from build123d import *

# Parameters (mm, degrees)
EXTRUDE_START       = -15
SKETCH_1_R          = 17
EXTRUDE_1_DEPTH     = 35
SKETCH_2_R          = 10
EXTRUDE_2_DEPTH     = 47
FILLET_3_R          = 3
FILLET_4_R          = 20
SKETCH_4_W          = 20
SKETCH_4_H          = 21.133558335
CUT_EXTRUDE_2_DEPTH = 35
SKETCH_5_R          = 4
CUT_EXTRUDE_3_DEPTH = 35
CUT_EXTRUDE_START   = 20
SKETCH_6_W          = 15
SKETCH_6_H          = 20.573480962
CUT_EXTRUDE_4_DEPTH = 4
CUT_EXTRUDE_START_2 = -20
SKETCH_7_W          = 20
SKETCH_7_H          = 18.159164137
CUT_EXTRUDE_5_DEPTH = 4
SKETCH_8_R          = 4
CUT_EXTRUDE_6_DEPTH = 35


with BuildPart() as part:
    # Эскиз1 → Вытянуть1 (new body)
    with BuildSketch(Plane(origin=(0, 0, 0), x_dir=(1, 0, 0), z_dir=(0, 1, 0)).offset(EXTRUDE_START)):
        with Locations(Location((0, 0, 0), (0, 0, 270))):
            Circle(SKETCH_1_R)
    extrude(amount=EXTRUDE_1_DEPTH)

    # Эскиз2 → Вытянуть2 (add)
    with BuildSketch(Plane.XZ.offset(15)):
        with Locations(Location((0, 0, 0), (0, 0, 90))):
            Circle(SKETCH_2_R)
    extrude(amount=EXTRUDE_2_DEPTH)

    # Скругление3
    fillet_3_edges = [part.edges().sort_by_distance(p)[0] for p in [
        (0, 20, -17),
    ]]
    fillet(fillet_3_edges, radius=FILLET_3_R)

    # Скругление4
    # the kernel refuses this fillet: 20 mm, written as the material it adds along each edge
    with BuildSketch(Plane(origin=(0, -15, 0), x_dir=(0, 0, 1), z_dir=(1, 0, 0))) as fillet_4_piece_1:
        with BuildLine():
            CenterArc((30, 15.198684154), FILLET_4_R, 180, 49.458398126)
            Line((10, 15.198684154), (9.6, 15.198684154))
            Line((9.6, 15.198684154), (9.6, 0))
            Line((9.6, 0), (10, -0.4))
            ThreePointArc((10, -0.4), (13.5, -0.4), (16.74, -0.303973683))
            Line((16.74, -0.303973683), (17, 0))
        make_face()
    revolve(axis=Axis((0, -15, 0), (0, -1, 0)))

    # Эскиз4 → Вырез-Вытянуть2 (cut, symmetric)
    with BuildSketch(Plane.XY):
        with Locations((0, 10.566779168)):
            Rectangle(SKETCH_4_W, SKETCH_4_H)
    extrude(amount=CUT_EXTRUDE_2_DEPTH, both=True, mode=Mode.SUBTRACT)

    # Эскиз5 → Вырез-Вытянуть3 (cut, symmetric)
    with BuildSketch(Plane(origin=(0, 0, 0), x_dir=(0, 0, -1), z_dir=(1, 0, 0))):
        with Locations((0, 11.128860454)):
            Circle(SKETCH_5_R)
    extrude(amount=CUT_EXTRUDE_3_DEPTH, both=True, mode=Mode.SUBTRACT)

    # Эскиз6 → Вырез-Вытянуть4 (cut)
    with BuildSketch(Plane(origin=(0, 0, 0), x_dir=(0, 0, -1), z_dir=(1, 0, 0)).offset(CUT_EXTRUDE_START)):
        with Locations((0, 10.338040732)):
            Rectangle(SKETCH_6_W, SKETCH_6_H)
    extrude(amount=-CUT_EXTRUDE_4_DEPTH, mode=Mode.SUBTRACT)

    # Эскиз7 → Вырез-Вытянуть5 (cut)
    with BuildSketch(Plane(origin=(0, 0, 0), x_dir=(0, 0, -1), z_dir=(1, 0, 0)).offset(CUT_EXTRUDE_START_2)):
        with Locations((0, 11.708442525)):
            Rectangle(SKETCH_7_W, SKETCH_7_H)
    extrude(amount=CUT_EXTRUDE_5_DEPTH, mode=Mode.SUBTRACT)

    # Эскиз8 → Вырез-Вытянуть6 (cut, symmetric)
    with BuildSketch(Plane(origin=(0, 0, 0), x_dir=(0, 0, -1), z_dir=(1, 0, 0))):
        with Locations((0.082515947, -53.926937182)):
            Circle(SKETCH_8_R)
    extrude(amount=CUT_EXTRUDE_6_DEPTH, both=True, mode=Mode.SUBTRACT)


solid = part.part
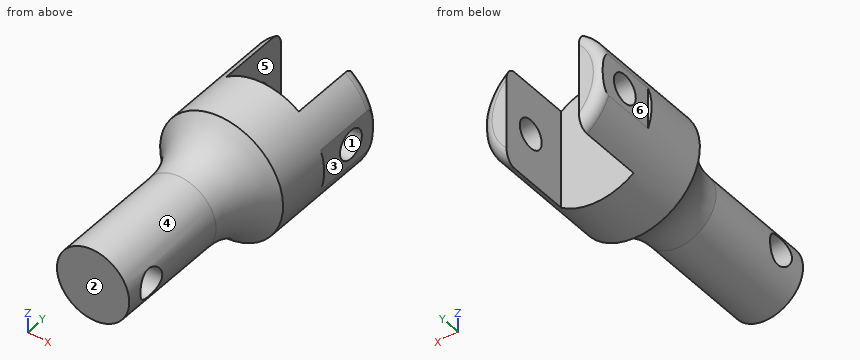
Can you work these out from the model? Positions are in its coordinate system, mm. Face numbers are marked on the shaded views. A direction names the side the tool comes from. Round coordinates to 2 decimals unless told otherwise and drop trailing zeros. Order: outer loops, then holes, each group sorted by start corner. A loop starts at its lowest first (then second) coordinate and runs counter-clockwise, first axis right, second up. Notation, with made-up numbers: (-24.75, -11) -> (-11.75, -11) arc R34 cw to (-11.75, 21) -> close; hole circle Ø9 at (-16.75, -8.75). An arc over 180 degrees is marked (long way). Write each question's results on one line, items separated by ' | '. Start each with the question number.
Item 1: If we section it at C-C, the plane z = 0: State how many separate pieces and enclosed holes the cut face has, then the cut area to 3 significant figures.
Item 2: Please list where these lines run through material, in increasing order: L1, parallel to X at y = -47, z = 0; L2, parallel to X at y = -41, z = 2; L3, parallel to X at y = 6, z = 11.
Item 3: Thinking about a two-plate mould opening in Y: for the marked faces 1, 2 and 3, which applies, +Y half, -Y half, draft (parallel to the pull), parting line (faces both ways), or undercut?
Item 4: If we section it at A-A, the plane x = 0: Write out the boundary of the cut face in (y, z).
Item 5: If we section it at D-D, the plane y = -33: Write out the boundary of the cut face in (x, z).
Item 6: If we section it at B-B, the plane y = 13.5: Write out the boundary of the cut face in (x, z), then the cut area to 3 significant figures.
Item 7: Will these pins go through, and if not, where does the flat tip stop? pin 1 (5.5 mm diameter, centred on y = 13, z = 0.5, fed in from -X); pin 2 (8 mm diameter, centred on x = 3, y = -35, fed in from -Z); pin 3 (1 mm diameter, centred on x = 12.5, y = -15.5, fed in from +Z).
Item 8: Which directions (+Z, -Z, +X, -X, +Y, -Y) give clear straight access to the entire face, cutting with the end or side of a thin tool? Please do the marked faces 4, 5 and 6.
Results:
1) separate pieces: 4 | enclosed holes: 0 | area: 1,500 mm2
2) L1: x = -10 to 10 | L2: x = -9.8 to 9.8 | L3: x = -12.96 to -10, 10 to 12.96
3) face 1: undercut | face 2: -Y half | face 3: draft
4) outline: (-62, -10) -> (-30.2, -10) arc R20 cw to (-15, -17) -> (0, -17) -> (0, 17) -> (-15, 17) arc R20 cw to (-30.2, 10) -> (-62, 10) -> close; hole circle Ø8 at (-53.93, -0.08)
5) outline: circle Ø20 at (0, 0)
6) outline: (-16, -5.74) arc R17 ccw to (-10, -13.75) -> (-10, -3.22) -> (-16, -3.22) -> close; (-16, 3.22) -> (-10, 3.22) -> (-10, 13.75) arc R17 ccw to (-16, 5.74) -> close; (10, -13.75) arc R17 ccw to (16, -5.74) -> (16, -3.22) -> (10, -3.22) -> close; (10, 3.22) -> (16, 3.22) -> (16, 5.74) arc R17 ccw to (10, 13.75) -> close | area: 177 mm2
7) pin 1: stops at x = -16 | pin 2: stops at z = -10 | pin 3: stops at z = 11.68
8) face 4: -Y | face 5: +Z, -Z, +Y | face 6: +Z, -Z, -X, +Y
